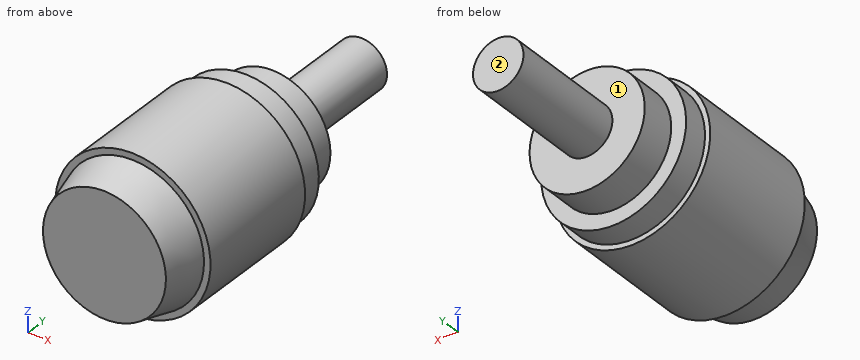
```python
from build123d import *

# Parameters (mm, degrees)
SKETCH_2_R      = 4.45
EXTRUDE_1_DEPTH = 2.8
SKETCH_3_R      = 1.95
EXTRUDE_2_DEPTH = 9.4


with BuildPart() as part:
    # 草图1 → 旋转1 (revolve)
    with BuildSketch(Plane.XY, mode=Mode.PRIVATE) as revolve_1_sk:
        Polygon((0, 0), (4.75, 0), (5.5, 3), (6, 3), (6, 13), (5.6, 13), (5.6, 15), (0, 15), align=None)
    revolve(revolve_1_sk.sketch.rotate(Axis((0, 15.733998589, 0), (0, -1, 0)), 90), axis=Axis((0, 15.733998589, 0), (0, -1, 0)))

    # 草图2 → 凸台-拉伸1 (add)
    with BuildSketch(Plane(origin=(0, 15, 0), x_dir=(1, 0, 0), z_dir=(0, 1, 0))):
        with Locations(Location((0, 0, 0), (0, 0, 270))):
            Circle(SKETCH_2_R)
    extrude(amount=EXTRUDE_1_DEPTH)

    # 草图3 → 凸台-拉伸2 (add)
    with BuildSketch(Plane(origin=(0, 17.8, 0), x_dir=(1, 0, 0), z_dir=(0, 1, 0))):
        with Locations(Location((0, 0, 0), (0, 0, 270))):
            Circle(SKETCH_3_R)
    extrude(amount=EXTRUDE_2_DEPTH)


solid = part.part
```
Can you work these out from the model? Positions are in its coordinate system, mm. Face numbers are marked on the shaded views. A direction names the side the tool comes from. Coordinates: 2 decimals unless noted, no trailing zeros. Write each loop counter-clockwise with the first axis right and the second up, starting at its lowest first coordinate (ties: lowest second). Pieces come first, ordered by that corner, then holes. Notation, with made-up numbers: M 81.5,9.5 L 95.5,9.5 A16 ccw 95.5,26.5 Z; hole C -38.5,-31 d9. An arc over 180 degrees is marked long. Answer as CSV lines item,"result".
Item 1: Imagine slicing it at D-D on y = 11.5. List the corners of the cut face in (x, z) for me, plus the area to 3 significant figures.
Geometry results:
outline,"C 0,0 d12"
area,"113 mm2"
Item 2: Please list where these lines run through material, in increasing order: line 1 along Y through (x, z) = (2.75, 2.5); line 2 along X through (y, z) = (10.5, 2.25); line 3 along Z through (x, y) = (-1.75, 23).
Geometry results:
line 1,"y = 0 to 17.8"
line 2,"x = -5.56 to 5.56"
line 3,"z = -0.86 to 0.86"
Item 3: Imagine slicing it at C-C on y = 19.75. List the corners of the cut face in (x, z) for me.
Geometry results:
outline,"C 0,0 d3.9"
Item 4: Imagine slicing it at B-B on z = 0. List the corners of the cut face in (x, y) for me, plus the area to 3 significant figures.
Geometry results:
outline,"M -6,3 L -5.5,3 L -4.75,0 L 4.75,0 L 5.5,3 L 6,3 L 6,13 L 5.6,13 L 5.6,15 L 4.45,15 L 4.45,17.8 L 1.95,17.8 L 1.95,27.2 L -1.95,27.2 L -1.95,17.8 L -4.45,17.8 L -4.45,15 L -5.6,15 L -5.6,13 L -6,13 Z"
area,"235 mm2"
Item 5: I'm going to push flat-ended pins straight in: P1, Ø5.5, axis at x = 2, z = 0, coming from the +Y side; P2, Ø1, axis at x = -3.5, z = -2.5, coming from the +Y side; P3, Ø3, axis at x = 4.5, y = 24, coming from the -Z side. Where does each tip first touch, or does it pass through?
Geometry results:
P1,"stops at y = 27.2"
P2,"stops at y = 17.8"
P3,"passes through"
Item 6: On a 3-axis mill with a long thin cutter (end or side, diameter ignored), from which of +Z, -Z, +X, -X, +Y, -Y can I reach the whole of each face in a straight line? I mean the marked faces 1 and 2. Say none if no direction works.
Geometry results:
face 1,"+Y"
face 2,"+Z, -Z, +X, -X, +Y"
Item 7: Imagine slicing it at A-A on x = 0. List the corners of the cut face in (y, z) for me, plus the area to 3 significant figures.
Geometry results:
outline,"M 0,-4.75 L 3,-5.5 L 3,-6 L 13,-6 L 13,-5.6 L 15,-5.6 L 15,-4.45 L 17.8,-4.45 L 17.8,-1.95 L 27.2,-1.95 L 27.2,1.95 L 17.8,1.95 L 17.8,4.45 L 15,4.45 L 15,5.6 L 13,5.6 L 13,6 L 3,6 L 3,5.5 L 0,4.75 Z"
area,"235 mm2"
